from build123d import *

# Parameters (mm, degrees)
EXTRUDE_1_DEPTH = 20
SKETCH_1_3_W    = 4
SKETCH_1_3_H    = 4
SKETCH_1_3_R    = 1
EXTRUDE_2_DEPTH = 6
EXTRUDE_START   = -3
SKETCH_1_4_W    = 4
SKETCH_1_4_H    = 4
SKETCH_1_4_R    = 1
SKETCH_1_4_W_2  = 12.937036518
SKETCH_1_4_H_2  = 3
EXTRUDE_3_DEPTH = 3
FILLET_1_R      = 2


with BuildPart() as part:
    # Sketch 1 → Extrude 1 (new body)
    with BuildSketch(Plane(origin=(0, 0, 0), x_dir=(1, 0, 0), z_dir=(0, 1, 0))):
        Polygon((-23, 6.5), (-23, 10.5), (-19, 10.5), (-6.718518259, 10.5), (-6.718518259, 13.5), (-26, 13.5), (-26, -13), (25.5, -13), (25.5, 13.5), (6.218518259, 13.5), (6.218518259, 10.5), (18.5, 10.5), (22.5, 10.5), (22.5, 6.5), (22.5, -6), (22.5, -10), (18.5, -10), (-19, -10), (-23, -10), (-23, -6), align=None)
    extrude(amount=EXTRUDE_1_DEPTH)

    # Sketch 1_3 → Extrude 2 (add)
    # profile 1 of 4: a face of its own
    with BuildSketch(Plane(origin=(0, 0, 0), x_dir=(1, 0, 0), z_dir=(0, 1, 0))):
        with Locations((-21, 8.5)):
            Rectangle(SKETCH_1_3_W, SKETCH_1_3_H)
        with Locations(Location((-21.5, 9, 0), (0, 0, 270))):
            Circle(SKETCH_1_3_R, mode=Mode.SUBTRACT)
    # profile 2 of 4: a face of its own
    with BuildSketch(Plane(origin=(0, 0, 0), x_dir=(1, 0, 0), z_dir=(0, 1, 0))):
        with Locations((20.5, 8.5)):
            Rectangle(SKETCH_1_3_W, SKETCH_1_3_H)
        with Locations(Location((21, 9, 0), (0, 0, 270))):
            Circle(SKETCH_1_3_R, mode=Mode.SUBTRACT)
    # profile 3 of 4: a face of its own
    with BuildSketch(Plane(origin=(0, 0, 0), x_dir=(1, 0, 0), z_dir=(0, 1, 0))):
        with Locations((20.5, -8)):
            Rectangle(SKETCH_1_3_W, SKETCH_1_3_H)
        with Locations(Location((21, -8.5, 0), (0, 0, 270))):
            Circle(SKETCH_1_3_R, mode=Mode.SUBTRACT)
    # profile 4 of 4: a face of its own
    with BuildSketch(Plane(origin=(0, 0, 0), x_dir=(1, 0, 0), z_dir=(0, 1, 0))):
        with Locations((-21, -8)):
            Rectangle(SKETCH_1_3_W, SKETCH_1_3_H)
        with Locations(Location((-21.5, -8.5, 0), (0, 0, 270))):
            Circle(SKETCH_1_3_R, mode=Mode.SUBTRACT)
    extrude(amount=EXTRUDE_2_DEPTH)

    # Sketch 1_4 → Extrude 3 (add)
    # profile 1 of 11: a face of its own
    with BuildSketch(Plane(origin=(0, 0, 0), x_dir=(1, 0, 0), z_dir=(0, 1, 0)).offset(EXTRUDE_START)):
        Polygon((-23, 6.5), (-23, 10.5), (-19, 10.5), (-6.718518259, 10.5), (-6.718518259, 13.5), (-26, 13.5), (-26, -13), (25.5, -13), (25.5, 13.5), (6.218518259, 13.5), (6.218518259, 10.5), (18.5, 10.5), (22.5, 10.5), (22.5, 6.5), (22.5, -6), (22.5, -10), (18.5, -10), (-19, -10), (-23, -10), (-23, -6), align=None)
    # profile 2 of 11: a face of its own
    with BuildSketch(Plane(origin=(0, 0, 0), x_dir=(1, 0, 0), z_dir=(0, 1, 0)).offset(EXTRUDE_START)):
        Polygon((-6.718518259, 10.5), (-19, 10.5), (-19, 6.5), (-23, 6.5), (-23, -6), (-19, -6), (-19, -10), (18.5, -10), (18.5, -6), (22.5, -6), (22.5, 6.5), (18.5, 6.5), (18.5, 10.5), (6.218518259, 10.5), align=None)
    # profile 3 of 11: a face of its own
    with BuildSketch(Plane(origin=(0, 0, 0), x_dir=(1, 0, 0), z_dir=(0, 1, 0)).offset(EXTRUDE_START)):
        with Locations((20.5, -8)):
            Rectangle(SKETCH_1_4_W, SKETCH_1_4_H)
        with Locations(Location((21, -8.5, 0), (0, 0, 270))):
            Circle(SKETCH_1_4_R, mode=Mode.SUBTRACT)
    # profile 4 of 11: a face of its own
    with BuildSketch(Plane(origin=(0, 0, 0), x_dir=(1, 0, 0), z_dir=(0, 1, 0)).offset(EXTRUDE_START)):
        with Locations((20.5, 8.5)):
            Rectangle(SKETCH_1_4_W, SKETCH_1_4_H)
        with Locations(Location((21, 9, 0), (0, 0, 270))):
            Circle(SKETCH_1_4_R, mode=Mode.SUBTRACT)
    # profile 5 of 11: a face of its own
    with BuildSketch(Plane(origin=(0, 0, 0), x_dir=(1, 0, 0), z_dir=(0, 1, 0)).offset(EXTRUDE_START)):
        with Locations((-21, -8)):
            Rectangle(SKETCH_1_4_W, SKETCH_1_4_H)
        with Locations(Location((-21.5, -8.5, 0), (0, 0, 270))):
            Circle(SKETCH_1_4_R, mode=Mode.SUBTRACT)
    # profile 6 of 11: a face of its own
    with BuildSketch(Plane(origin=(0, 0, 0), x_dir=(1, 0, 0), z_dir=(0, 1, 0)).offset(EXTRUDE_START)):
        with Locations(Location((-21.5, -8.5, 0), (0, 0, 270))):
            Circle(SKETCH_1_4_R)
    # profile 7 of 11: a face of its own
    with BuildSketch(Plane(origin=(0, 0, 0), x_dir=(1, 0, 0), z_dir=(0, 1, 0)).offset(EXTRUDE_START)):
        with Locations((-21, 8.5)):
            Rectangle(SKETCH_1_4_W, SKETCH_1_4_H)
        with Locations(Location((-21.5, 9, 0), (0, 0, 270))):
            Circle(SKETCH_1_4_R, mode=Mode.SUBTRACT)
    # profile 8 of 11: a face of its own
    with BuildSketch(Plane(origin=(0, 0, 0), x_dir=(1, 0, 0), z_dir=(0, 1, 0)).offset(EXTRUDE_START)):
        with Locations(Location((-21.5, 9, 0), (0, 0, 270))):
            Circle(SKETCH_1_4_R)
    # profile 9 of 11: a face of its own
    with BuildSketch(Plane(origin=(0, 0, 0), x_dir=(1, 0, 0), z_dir=(0, 1, 0)).offset(EXTRUDE_START)):
        with Locations(Location((21, 9, 0), (0, 0, 270))):
            Circle(SKETCH_1_4_R)
    # profile 10 of 11: a face of its own
    with BuildSketch(Plane(origin=(0, 0, 0), x_dir=(1, 0, 0), z_dir=(0, 1, 0)).offset(EXTRUDE_START)):
        with Locations(Location((21, -8.5, 0), (0, 0, 270))):
            Circle(SKETCH_1_4_R)
    # profile 11 of 11: a face of its own
    with BuildSketch(Plane(origin=(0, 0, 0), x_dir=(1, 0, 0), z_dir=(0, 1, 0)).offset(EXTRUDE_START)):
        with Locations((-0.25, 12)):
            Rectangle(SKETCH_1_4_W_2, SKETCH_1_4_H_2)
    extrude(amount=EXTRUDE_3_DEPTH)

    # Fillet 1
    fillet_1_edges = [part.edges().sort_by_distance(p)[0] for p in [
        (25.5, 8.5, 13),
        (-26, 8.5, 13),
        (-26, 8.5, -13.5),
        (25.5, 8.5, -13.5),
        (-16.359259129, 20, -13.5),
        (-26, 20, -0.25),
        (-0.25, 20, 13),
        (25.5, 20, -0.25),
        (15.859259129, 20, -13.5),
    ]]
    fillet(fillet_1_edges, radius=FILLET_1_R)


solid = part.part
Source: CAD feature listing. Evaluate the final solid. Frame: model axes, mm. A direction names the side the tool comes from. Round coordinates to 2 decimals unless told otherwise and drop trailing zeros. Loops run counter-clockwise (first coordinate to the right, second up) from the corner with the lowest first, then second, coordinate; pieces in that order, holes last. Notation, with made-up numbers: (-39, 80) -> (-9, 80) arc R10 ccw to (-9, 94) -> close; hole circle Ø10 at (-33.75, -29.5). An arc over 180 degrees is marked (long way). Answer as a JSON object with one key per item and string values. Group by question number.
Q1. Section query D-D (z = -9.5). Output: boundary loops of the cut face in (x, y).
Q2. Access query for faces 1 (the flat face through (-1, -3, 0)), 2 (the flat face through (-6.719, 10, -12)), 3 (the flat face through (-15, 10, -10.5)). Directions: +Z, -Z, +X, -X, +Y, -Y. A direction counts if a zero-diameter tool reaches every point of the face in a straight line with its end or side. Return the directions, or none.
Q3. Contact query for flat-ended pins moving along their axis: P1, Ø2.5, axis at x = 21, z = 8.5, coming from the +Y side; P2, Ø10, axis at x = -0.5, z = -6, coming from the +Y side. Output: stop coordinate, or through.
Q4. Ray query, line 1 (X direction, y = 2.2, z = 8.5); line 2 (Z direction, x = -12.5, y = 6.25); line 3 (X direction, y = 7.75, z = -4.75). Return the intervals inside material, ascending. Write a range as from..to.
Q5. Section query C-C (x = 19.5). Output: boundary loops of the cut face in (y, z).
Q6. Section query A-A (y = 17.5). Output: boundary loops of the cut face in (x, z), plus the area to 3 significant figures.
Q7. Section query B-B (z = 6.75). Output: boundary loops of the cut face in (x, y).
Q8. Mould query, pull axis X, two halves, no side actions, for faces 4 (the flat face through (20, 6, 7.5)), 5 (the flat face through (0, -2, -13.5)), 6 (the flat face through (0, 10, 10)), 7 (the cylindrical face through (-25.4, 7.65, -12.93)). Classes: pulls with the +X half, pulls with the -X half, needs draft (parallel to the pull), parting line crosses it, or undercut.
Completed:
{
 "1": {"outline": "(-26, -3) -> (25.5, -3) -> (25.5, 18) arc R2 ccw to (23.5, 20) -> (22.5, 20) -> (22.5, 6) -> (21.87, 6) -> (21.87, 0) -> (20.13, 0) -> (20.13, 6) -> (18.5, 6) -> (18.5, 0) -> (-19, 0) -> (-19, 6) -> (-20.63, 6) -> (-20.63, 0) -> (-22.37, 0) -> (-22.37, 6) -> (-23, 6) -> (-23, 20) -> (-24, 20) arc R2 ccw to (-26, 18) -> close"},
 "2": {"face 1": "+Z, -Z, +X, -X, -Y", "face 2": "-Z, +Y", "face 3": "+Y"},
 "3": {"P1": "y = 6", "P2": "y = 0"},
 "4": {"line 1": "-26..-22.5, -20.5..-19, 18.5..20, 22..25.5", "line 2": "-13.5..-10.5, 10..13", "line 3": "-26..-23, 22.5..25.5"},
 "5": {"outline": "(-3, -13.5) -> (18, -13.5) arc R2 ccw to (20, -11.5) -> (20, -10.5) -> (6, -10.5) -> (6, -6.5) -> (0, -6.5) -> (0, 6) -> (6, 6) -> (6, 10) -> (20, 10) -> (20, 11) arc R2 ccw to (18, 13) -> (-3, 13) -> close"},
 "6": {"outline": "(-26, -11.5) arc R2 ccw to (-24, -13.5) -> (-6.72, -13.5) -> (-6.72, -10.5) -> (-23, -10.5) -> (-23, 10) -> (22.5, 10) -> (22.5, -10.5) -> (6.22, -10.5) -> (6.22, -13.5) -> (23.5, -13.5) arc R2 ccw to (25.5, -11.5) -> (25.5, 11) arc R2 ccw to (23.5, 13) -> (-24, 13) arc R2 ccw to (-26, 11) -> close", "area": "390 mm²"},
 "7": {"outline": "(-26, -3) -> (25.5, -3) -> (25.5, 18) arc R2 ccw to (23.5, 20) -> (22.5, 20) -> (22.5, 6) -> (18.5, 6) -> (18.5, 0) -> (-19, 0) -> (-19, 6) -> (-23, 6) -> (-23, 20) -> (-24, 20) arc R2 ccw to (-26, 18) -> close"},
 "8": {"face 4": "undercut", "face 5": "needs draft", "face 6": "undercut", "face 7": "pulls with the -X half"}
}
